from build123d import *

# Parameters (mm, degrees)
SKETCH1_W           = 1
SKETCH1_H           = 10
BOSS_EXTRUDE1_DEPTH = 3


with BuildPart() as part:
    # Sketch1 → Boss-Extrude1 (new body)
    with BuildSketch(Plane.XY):
        Polygon((1, 10), (1, 0), (18, 0), (18, 40), (15, 40), (5, 40), (1, 40), (1, 30), (1, 20), align=None)
        Polygon((18, 40), (18, 0), (35, 0), (35, 10), (35, 20), (35, 30), (35, 40), (31, 40), (21, 40), align=None)
        with Locations((0.5, 5)):
            Rectangle(SKETCH1_W, SKETCH1_H)
        with Locations((0.5, 25)):
            Rectangle(SKETCH1_W, SKETCH1_H)
        with Locations((35.5, 25)):
            Rectangle(SKETCH1_W, SKETCH1_H)
        with Locations((35.5, 5)):
            Rectangle(SKETCH1_W, SKETCH1_H)
        Polygon((0, 43), (0, 40), (1, 40), (5, 40), (5, 43), align=None)
        Polygon((15, 40), (18, 40), (21, 40), (21, 43), (15, 43), align=None)
        Polygon((31, 43), (31, 40), (35, 40), (36, 40), (36, 43), align=None)
    extrude(amount=BOSS_EXTRUDE1_DEPTH)


solid = part.part
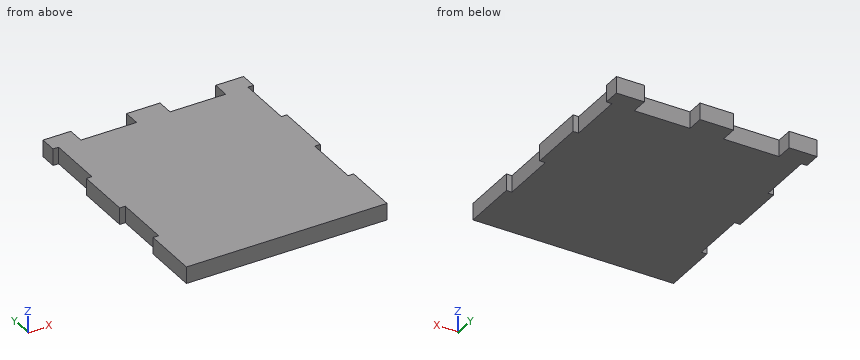
Read the model definition and answer for the solid it produces. Units are mm, in the model's axes. Round coordinates to 2 decimals unless told otherwise and drop trailing zeros. Order: outer loops, then holes, each group sorted by start corner. A loop starts at its lowest first (then second) coordinate and runs counter-clockwise, first axis right, second up.
1) Straight lines are drawn through the part: L1, parallel to X at y = 30.5, z = 2.8; L2, parallel to Y at x = 24, z = 2.9. For each, find the intervals that lie inside material, in ascending order.
2) The part is cut by section A-A on z = 1.9. Write down the section's boundary in (x, y), plus the area to 3 significant figures.
3) The part is cut by section B-B on y = 32.5. Write down the section's boundary in (x, z).
4) Flat-ended cylindrical pins translate along their axes: pin 1 (1.5 mm diameter, centred on x = 6.5, z = 0.5, fed in from +Y); pin 2 (1 mm diameter, centred on y = 36.5, z = 2, fed in from +X). Find the tip coordinate at first contact, or state that the pin passes through.
5) The part is cut by section C-C on x = 24. Write down the section's boundary in (y, z).
Resolved:
1. L1: x = 1 to 35
1. L2: y = 0 to 40
2. outline: (0, 0) - (36, 0) - (36, 10) - (35, 10) - (35, 20) - (36, 20) - (36, 30) - (35, 30) - (35, 40) - (36, 40) - (36, 43) - (31, 43) - (31, 40) - (21, 40) - (21, 43) - (15, 43) - (15, 40) - (5, 40) - (5, 43) - (0, 43) - (0, 40) - (1, 40) - (1, 30) - (0, 30) - (0, 20) - (1, 20) - (1, 10) - (0, 10) - close
2. area: 1,450 mm2
3. outline: (1, 0) - (35, 0) - (35, 3) - (1, 3) - close
4. pin 1: stops at y = 40
4. pin 2: stops at x = 35
5. outline: (0, 0) - (40, 0) - (40, 3) - (0, 3) - close
